```python
from build123d import *

# Parameters (mm, degrees)
SKETCH1_R                 = 18.26006
BOSS_EXTRUDE1_DEPTH       = 5.08
F_4_CLEARANCE_HOLE1_D     = 3.302
F_4_CLEARANCE_HOLE2_D     = 9.525
F_4_CLEARANCE_HOLE2_DEPTH = 57.15
F_4_CLEARANCE_HOLE2_TIP   = 2.861598698


with BuildPart() as part:
    # Sketch1 → Boss-Extrude1 (new body)
    with BuildSketch(Plane(origin=(0, 0, 0), x_dir=(0, 0, -1), z_dir=(1, 0, 0))):
        Circle(SKETCH1_R)
    extrude(amount=BOSS_EXTRUDE1_DEPTH)

    # #4 Clearance Hole1 (through all)
    with Locations(Plane(origin=(5.08, 0, 0), x_dir=(0, 0, -1), z_dir=(1, 0, 0))):
        with Locations((0, 7.9375), (6.874076643, 3.96875), (6.874076643, -3.96875), (0, -7.9375), (-6.874076643, -3.96875), (-6.874076643, 3.96875), (0, 0)):
            Hole(F_4_CLEARANCE_HOLE1_D / 2)

    # #4 Clearance Hole2
    with Locations(Plane(origin=(5.08, 0, 0), x_dir=(0, 0, -1), z_dir=(1, 0, 0))):
        with Locations((0, 0)):
            Hole(F_4_CLEARANCE_HOLE2_D / 2, depth=F_4_CLEARANCE_HOLE2_DEPTH)
            with Locations((0, 0, -(F_4_CLEARANCE_HOLE2_DEPTH + F_4_CLEARANCE_HOLE2_TIP / 2))):  # 118° drill point
                Cone(0, F_4_CLEARANCE_HOLE2_D / 2, F_4_CLEARANCE_HOLE2_TIP, mode=Mode.SUBTRACT)


solid = part.part
```
Geometry check sheet. Reference: the model listing, model coordinates, mm. Give positions to 0.01 mm unless a question says otherwise; leave off trailing zeros. Loops run counter-clockwise (first coordinate to the right, second up) from the corner with the lowest first, then second, coordinate; pieces in that order, holes last. Notation, with made-up numbers: M 82.25,-12.5 L 112.25,-12.5 A17 cw 112.25,5.5 Z; hole C 21,55.25 d7. An arc over 180 degrees is marked long. Write item = value, one per line. Start each with the question number.
1. Thickness scan on probe 1 along Y at (x, z) = (1.9, 0); probe 2 along Y at (x, z) = (1.5, -7.5); probe 3 along Z at (x, y) = (0.75, -6.5). Record the ranges inside material, lowest first.
2. Section check A-A, the plane z = 0. Enter the section's corners in (x, y).
3. Go/stop test with flat-tipped pins: P1, Ø5.5, axis at y = 3.97, z = -6.87, coming from the +X side; P2, Ø1.5, axis at x = 4, z = -2, coming from the -Y side; P3, Ø1.5, axis at x = 4.5, z = -0.5, coming from the +Y side; P4, Ø1.5, axis at x = 2.5, z = 7, coming from the +Y side. Record where each tip stops, or that it passes through.
4. Section check C-C, the plane x = 3.3. Enter the section's corners in (y, z) (1 decimal).
5. Section check D-D, the plane z = -4. Enter the section's corners in (x, y).
6. Draft check along Z on faces 1 (the face through (0, -4, -4)), 2 (the face through (2.5, 5.48, -17.42)), 3 (the face through (2.504, -4.973, -8.184)). Enter one of: +Z half, -Z half, draft (parallel to the pull), parting line (faces both ways), or undercut.
7. Section check B-B, the plane y = 0. Enter the section's corners in (x, z).
Values follow:
q1.probe_1 = -18.26 to -9.59, -6.29 to -4.76, 4.76 to 6.29, 9.59 to 18.26
q1.probe_2 = -16.65 to -5.5, -2.44 to 2.44, 5.5 to 16.65
q1.probe_3 = -17.06 to -0.81, 0.81 to 17.06
q2.outline = M 0,-18.26 L 5.08,-18.26 L 5.08,-9.59 L 0,-9.59 Z; M 0,-6.29 L 5.08,-6.29 L 5.08,-4.76 L 0,-4.76 Z; M 0,4.76 L 5.08,4.76 L 5.08,6.29 L 0,6.29 Z; M 0,9.59 L 5.08,9.59 L 5.08,18.26 L 0,18.26 Z
q3.P1 = 5.08
q3.P2 = -18.22
q3.P3 = 18.26
q3.P4 = 17.16
q4.outline = C 0,0 d36.5; hole C -7.9,0 d3.3; hole C -4,-6.9 d3.3; hole C -4,6.9 d3.3; hole C 0,0 d9.5; hole C 4,-6.9 d3.3; hole C 4,6.9 d3.3; hole C 7.9,0 d3.3
q5.outline = M 0,-17.82 L 5.08,-17.82 L 5.08,-2.58 L 0,-2.58 Z; M 0,2.58 L 5.08,2.58 L 5.08,17.82 L 0,17.82 Z
q6.face_1 = draft
q6.face_2 = parting line
q6.face_3 = undercut
q7.outline = M 0,-18.26 L 5.08,-18.26 L 5.08,-4.76 L 0,-4.76 Z; M 0,4.76 L 5.08,4.76 L 5.08,18.26 L 0,18.26 Z
